```python
from build123d import *

# Parameters (mm, degrees)
CROQUIS1_R              = 61.885645
SALIENTE_EXTRUIR1_DEPTH = 8
CROQUIS2_R              = 20
CORTAR_EXTRUIR1_DEPTH   = 8
CROQUIS3_R              = 20
SALIENTE_EXTRUIR2_DEPTH = 4
CROQUIS4_R              = 19
SALIENTE_EXTRUIR3_DEPTH = 8.1661
CROQUIS5_R              = 1.25
CORTAR_EXTRUIR2_DEPTH   = 8.1661
CROQUIS6_R              = 1.25
CORTAR_EXTRUIR3_DEPTH   = 8.1661
CROQUIS7_R              = 19
CORTAR_EXTRUIR4_DEPTH   = 4.43


with BuildPart() as part:
    # Croquis1 → Saliente-Extruir1 (new body)
    with BuildSketch(Plane(origin=(0, 0, 0), x_dir=(1, 0, 0), z_dir=(0, 1, 0))):
        Circle(CROQUIS1_R)
    extrude(amount=SALIENTE_EXTRUIR1_DEPTH)

    # Croquis2 → Cortar-Extruir1 (cut)
    with BuildSketch(Plane(origin=(0, 8, 0), x_dir=(1, 0, 0), z_dir=(0, 1, 0))):
        Circle(CROQUIS2_R)
    extrude(amount=-CORTAR_EXTRUIR1_DEPTH, mode=Mode.SUBTRACT)

    # Croquis3 → Saliente-Extruir2 (add)
    with BuildSketch(Plane(origin=(0, 8, 0), x_dir=(1, 0, 0), z_dir=(0, 1, 0))):
        Circle(CROQUIS3_R)
    extrude(amount=-SALIENTE_EXTRUIR2_DEPTH)

    # Croquis4 → Saliente-Extruir3 (add)
    with BuildSketch(Plane(origin=(0, 4, 0), x_dir=(-1, 0, 0), z_dir=(0, -1, 0))):
        Circle(CROQUIS4_R)
    extrude(amount=-SALIENTE_EXTRUIR3_DEPTH)

    # Croquis5 → Cortar-Extruir2 (cut)
    with BuildSketch(Plane(origin=(0, 12.1661, 0), x_dir=(1, 0, 0), z_dir=(0, 1, 0))):
        with Locations((11.691342951, 6.75)):
            Circle(CROQUIS5_R)
        with Locations((0, 13.5)):
            Circle(CROQUIS5_R)
        with Locations((-11.691342951, 6.75)):
            Circle(CROQUIS5_R)
        with Locations((-11.691342951, -6.75)):
            Circle(CROQUIS5_R)
        with Locations((0, -13.5)):
            Circle(CROQUIS5_R)
        with Locations((11.691342951, -6.75)):
            Circle(CROQUIS5_R)
    extrude(amount=-CORTAR_EXTRUIR2_DEPTH, mode=Mode.SUBTRACT)

    # Croquis6 → Cortar-Extruir3 (cut)
    with BuildSketch(Plane(origin=(0, 12.1661, 0), x_dir=(1, 0, 0), z_dir=(0, 1, 0))):
        Circle(CROQUIS6_R)
    extrude(amount=-CORTAR_EXTRUIR3_DEPTH, mode=Mode.SUBTRACT)

    # Croquis7 → Cortar-Extruir4 (cut)
    with BuildSketch(Plane(origin=(0, 12.1661, 0), x_dir=(1, 0, 0), z_dir=(0, 1, 0))):
        Circle(CROQUIS7_R)
    extrude(amount=-CORTAR_EXTRUIR4_DEPTH, mode=Mode.SUBTRACT)


solid = part.part
```
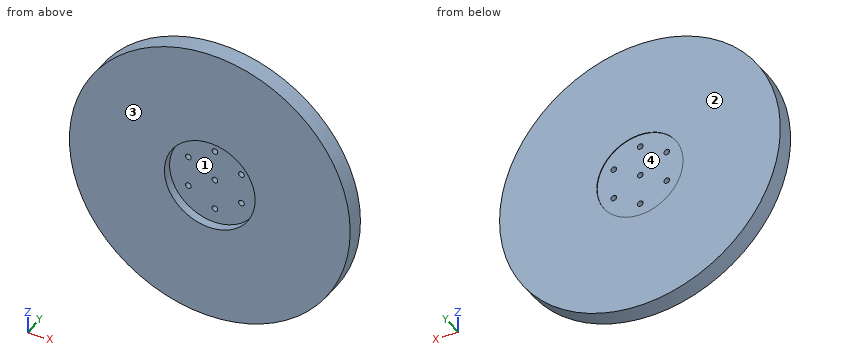
CAD build for the part. Positions are in the model's coordinates, mm. Face numbers are marked on the shaded views. A direction names the side the tool comes from. Give positions to 0.01 mm unless a question says otherwise; leave off trailing zeros. Order: outer loops, then holes, each group sorted by start corner. A loop starts at its lowest first (then second) coordinate and runs counter-clockwise, first axis right, second up.
(1) Flat gauge pins, fed straight in: pin 1 (3 mm diameter, centred on x = 11.69, z = -6.75, fed in from -Y); pin 2 (1.5 mm diameter, centred on y = 7, z = -31.5, fed in from +X); pin 3 (5 mm diameter, centred on x = 44.5, z = 19, fed in from -Y); pin 4 (2 mm diameter, centred on y = 1, z = -1.5, fed in from -X). Where does each tip first touch, or does it go through?
(2) Saw through at D-D, the plane z = -23.5. Give the cut face in (x, y), then the cut area to 3 significant figures.
(3) Saw through at B-B, the plane y = 1.5. Give the cut face in (x, z), then the cut area to 3 significant figures.
(4) Saw through at A-A, the plane x = 17.5. Give the cut face in (y, z).
(5) Tool access for the marked faces 3 and 4: list every direction of +Z, -Z, +X, -X, +Y, -Y with a clear straight run to the whole face (end or side of a thin tool).
(6) Drill centre lines: L1, parallel to X at y = 5.7, z = 0; L2, parallel to Z at x = -12.5, y = 4.5; L3, parallel to X at y = 6.4, z = -6.75. Where is each one in solid material? Low to high.
(7) Mould opens along X. For the marked faces 1 and 2 say: released by +X, released by -X, zero draft, split by the parting line, or undercut.
(8) Saw through at C-C, the plane z = 22. Give the cut face in (x, y).
Results found:
1. pin 1: stops at y = 4
1. pin 2: stops at x = 53.71
1. pin 3: stops at y = 0
1. pin 4: stops at x = -61.88
2. outline: (-57.25, 0) - (57.25, 0) - (57.25, 8) - (-57.25, 8) - close
2. area: 916 mm2
3. outline: circle Ø123.77 at (0, 0); hole circle Ø40 at (0, 0)
3. area: 10,800 mm2
4. outline: (0, -59.36) - (8, -59.36) - (8, -7.4) - (7.74, -7.4) - (7.74, 7.4) - (8, 7.4) - (8, 59.36) - (0, 59.36) - (0, 9.68) - (4, 9.68) - (4, -9.68) - (0, -9.68) - close
5. face 3: +Z, -Z, +X, -X, -Y
5. face 4: +Y
6. L1: x = -61.89 to -1.25, 1.25 to 61.89
6. L2: z = -60.61 to -7.7, -5.8 to 5.8, 7.7 to 60.61
6. L3: x = -61.52 to -12.94, -10.44 to 10.44, 12.94 to 61.52
7. face 1: undercut
7. face 2: zero draft
8. outline: (-57.84, 0) - (57.84, 0) - (57.84, 8) - (-57.84, 8) - close
